Build history of the part. All positions in model axes, mm. Face numbers are marked on the shaded views. A direction names the side the tool comes from. Round coordinates to 2 decimals unless told otherwise and drop trailing zeros. Write each loop counter-clockwise with the first axis right and the second up, starting at its lowest first coordinate (ties: lowest second). Pieces come first, ordered by that corner, then holes. Notation, with made-up numbers: (-24.75, -7) -> (2.25, -7) arc R26 ccw to (2.25, 28) -> close; hole circle Ø8 at (49.5, -14). An arc over 180 degrees is marked (long way). Return JSON: item names as keys, results as strings.
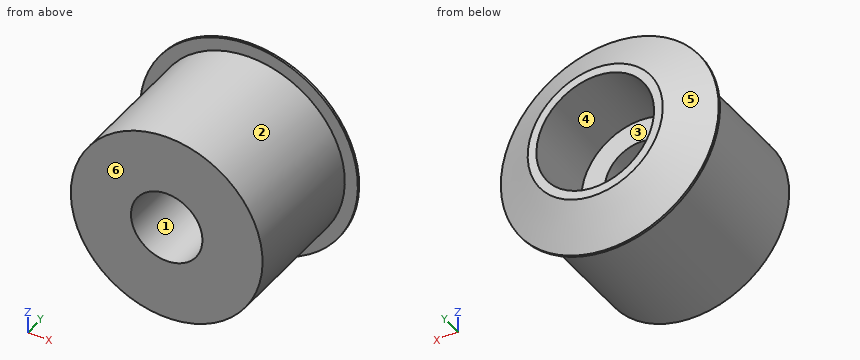
from build123d import *


with BuildPart() as part:
    # Esquisse1 → Révolution1 (revolve)
    with BuildSketch(Plane.XY, mode=Mode.PRIVATE) as r_volution1_sk:
        Polygon((4.1, 0), (4.1, 9.992413779), (6.75, 9.992413779), (6.75, 18.492413779), (7.75, 18.492413779), (12.5, 15.75), (12.5, 15.5), (11, 15.5), (11, 0), align=None)
    revolve(r_volution1_sk.sketch.rotate(Axis((0, 10.730531249, 0), (0, -1, 0)), 90), axis=Axis((0, 10.730531249, 0), (0, -1, 0)))  # turned: the seam where the file's is


solid = part.part
Q1. Saw through at A-A on x = 0. List the corners of the cut face in (y, z), then the cut area to 3 significant figures.
Verdict:
{"outline": "(0, -11) -> (15.5, -11) -> (15.5, -12.5) -> (15.75, -12.5) -> (18.49, -7.75) -> (18.49, -6.75) -> (9.99, -6.75) -> (9.99, -4.1) -> (0, -4.1) -> close; (0, 4.1) -> (9.99, 4.1) -> (9.99, 6.75) -> (18.49, 6.75) -> (18.49, 7.75) -> (15.75, 12.5) -> (15.5, 12.5) -> (15.5, 11) -> (0, 11) -> close", "area": "206 mm²"}
Q2. Saw through at C-C on y = 6. List the corners of the cut face in (x, z).
Verdict:
{"outline": "circle Ø22 at (0, 0); hole circle Ø8.2 at (0, 0)"}
Q3. Saw through at B-B on z = 0. List the corners of the cut face in (x, y).
Verdict:
{"outline": "(-12.5, 15.5) -> (-11, 15.5) -> (-11, 0) -> (-4.1, 0) -> (-4.1, 9.99) -> (-6.75, 9.99) -> (-6.75, 18.49) -> (-7.75, 18.49) -> (-12.5, 15.75) -> close; (4.1, 0) -> (11, 0) -> (11, 15.5) -> (12.5, 15.5) -> (12.5, 15.75) -> (7.75, 18.49) -> (6.75, 18.49) -> (6.75, 9.99) -> (4.1, 9.99) -> close"}
Q4. Wall check: L1, parallel to X at y = 2.5, z = 0; L2, parallel to Y at x = -4.25, z = -2; L3, parallel to X at y = 14.5, z = 0. Give the ranges that are in metal, low to high.
Verdict:
{"L1": "x = -11 to -4.1, 4.1 to 11", "L2": "y = 0 to 9.99", "L3": "x = -11 to -6.75, 6.75 to 11"}
Q5. Saw through at D-D on y = 12. List the corners of the cut face in (x, z).
Verdict:
{"outline": "circle Ø22 at (0, 0); hole circle Ø13.5 at (0, 0)"}
Q6. Two-plate mould, pull along X, no slides. Class the marked faces 4, 5 and 6: +X half, -X half, draft (parallel to the pull), parting line (faces both ways), or undercut.
Verdict:
{"face 4": "undercut", "face 5": "parting line", "face 6": "draft"}
Q7. 3-axis set-ups, long thin cutter, end or side, ignore diameter. For the marked faces 1, 2 and 3: which of +Z, -Z, +X, -X, +Y, -Y reach the whole face in a straight line?
Verdict:
{"face 1": "+Y, -Y", "face 2": "-Y", "face 3": "+Y"}
Q8. Pin check, flat tips, straight feed: pin 1 Ø6 at (x, y) = (-1, 8) entering from +Z; pin 2 Ø1.5 at (y, z) = (4.5, 8.5) entering from +X; pin 3 Ø13 at (x, z) = (0, 0) entering from -Y; pin 4 Ø5 at (y, z) = (4.5, 9.5) entering from -X. Stop position of each tip, or through.
Verdict:
{"pin 1": "stops at z = 11", "pin 2": "stops at x = 7.81", "pin 3": "stops at y = 0", "pin 4": "stops at x = -8.49"}
